Build history of the part. All positions in model axes, mm. Round coordinates to 2 decimals unless told otherwise and drop trailing zeros. Write each loop counter-clockwise with the first axis right and the second up, starting at its lowest first coordinate (ties: lowest second). Pieces come first, ordered by that corner, then holes. Notation, with made-up numbers: M 23,78.5 L 53,78.5 A14 ccw 53,95.5 Z; hole C 16.25,34.5 d6. An arc over 180 degrees is marked long. Write item = value, one per line. Start each with the question number.
Q1. Pull direction Y, two halves, no side cores. Call faces 1 (the flat face through (30, 65, -65)), 2 (the cylindrical face through (14.79, -128.18, 50.64)), 3 (the cylindrical face through (14.79, -19.527, -148.724)): released by +Y, released by -Y, zero draft, split by the parting line, or undercut.
Q2. Band-saw the part on A-A on z = 0. Write the cut outline in (x, y).
Q3. Band-saw the part on C-C on z = -109. Write the cut outline in (x, y).
Q4. Band-saw the part on D-D on y = 43. Write the cut outline in (x, z).
Q5. Probe L1, parallel to Y at x = 2, z = 124; L2, parallel to Z at x = 14, y = 40; L3, parallel to Z at x = 6.5, y = 52.5. List the from-to ranges inside material, lowest first.
Q6. Drop flat-ended pins along their axis: P1, Ø6, axis at x = 25, y = 107.5, coming from the -Z side; P2, Ø5, axis at x = 20.5, y = 23, coming from the -Z side; P3, Ø1.5, axis at x = 22, y = -81, coming from the -Z side. Give the stop position or say it passes through.
Autodesk Inventor part; units mm, degrees
ref_plane "YZ Plane" through (0, 0, 0) normal (1, 0, 0) x (0, 1, 0)
ref_plane "XZ Plane" through (0, 0, 0) normal (0, 1, 0) x (-1, 0, 0)
ref_plane "XY Plane" through (0, 0, 0) normal (0, 0, 1) x (1, 0, 0)
sketch "Sketch1" plane through (0, 0, 0) normal (0, 0, 1) x (1, 0, 0)
  line L0 (30, 150) -> (0, 150)
  line L1 (0, 150) -> (0, 85.25)
  line L2 (0, 85.25) -> (0, 0) construction
  line L3 (0, 0) -> (30, 0) construction
  line L4 (30, 150) -> (30, 85.25)
  line L5 (30, 85.25) -> (0, 85.25)
  line L6 (30, 85.25) -> (30, 0) construction
  dimension "d0" = 300
  dimension "d1" = 30
  dimension "d5" = 170.5
revolve "Revolution1" add sketch "Sketch1" angle 360 about axis through (0, 0, 0) along (1, 0, 0)
sketch "Sketch2" plane through (0, 0, 0) normal (-1, 0, 0) x (0, 0, 1)
  circle A0 centre (0, 0) radius 85.25
  line L0 (0, 125) -> (0, 0) construction
  circle A1 centre (0, 0) radius 150
  circle A2 centre (0, 0) radius 125 construction
  line L1 (0, 0) -> (47.8354, 115.4849) construction
  circle A3 centre (47.8354, 115.4849) radius 13
  dimension "d6" = 26
  dimension "d7" = 125
  dimension "d8" = 22.5
extrude "Extrusion1" cut sketch "Sketch2" against normal through all contours A3
pattern_circular "Circular Pattern1" count 8 over 360 about axis through (15, 0, 0) along (1, 0, 0) of "Extrusion1"
equation "\"d6\" = dd2"
equation "\"d7\" = 0.5 * k"
equation "\"d0\" = D"
equation "\"d1\" = b"
equation "\"d5\" = dd5"
equation "\"b\" = 30"
equation "\"D\" = 300"
equation "\"dd2\" = 26"
equation "\"dd5\" = 170.5"
equation "\"Size_Designation\" = 1.2345"
properties part number "DIN EN 1092-1 Plate Flange for Welding Type 01 - PN 25 150 x 168.3" material "Steel"
Conclusion:
q1.face_1 = zero draft
q1.face_2 = undercut
q1.face_3 = split by the parting line
q2.outline = M 0,-150 L 30,-150 L 30,-85.25 L 0,-85.25 Z; M 0,85.25 L 30,85.25 L 30,150 L 0,150 Z
q3.outline = M 0,-103.05 L 30,-103.05 L 30,-59.1 L 0,-59.1 Z; M 0,-36.57 L 30,-36.57 L 30,36.57 L 0,36.57 Z; M 0,59.1 L 30,59.1 L 30,103.05 L 0,103.05 Z
q4.outline = M 0,-143.7 L 30,-143.7 L 30,-127.55 L 0,-127.55 Z; M 0,-103.42 L 30,-103.42 L 30,-73.61 L 0,-73.61 Z; M 0,73.61 L 30,73.61 L 30,103.42 L 0,103.42 Z; M 0,127.55 L 30,127.55 L 30,143.7 L 0,143.7 Z
q5.L1 = -84.4 to -57.66, -38.01 to 38.01, 57.66 to 84.4
q5.L2 = -144.57 to -125.86, -105.11 to -75.28, 75.28 to 105.11, 125.86 to 144.57
q5.L3 = -140.51 to -127.62, -103.35 to -67.17, 67.17 to 103.35, 127.62 to 140.51
q6.P1 = -107.61
q6.P2 = -148.59
q6.P3 = -126.73
